from build123d import *
from build123d.topology import SkipClean

# Parameters (mm, degrees)
SKETCH_1_R      = 1.25
EXTRUDE_1_DEPTH = 2.5
FILLET_1_R      = 2
SKETCH_2_R      = 4.625
EXTRUDE_2_DEPTH = 13.7
SKETCH_3_R      = 1
EXTRUDE_3_DEPTH = 5.5
EXTRUDE_4_DEPTH = 2
EXTRUDE_START   = 11.3
SKETCH_5_R      = 13.75
EXTRUDE_5_DEPTH = 11.3
FILLET_2_R      = 4


with BuildPart() as part:
    # 草图1 → 凸台-拉伸1 (new body)
    with BuildSketch(Plane(origin=(0, 0, 0), x_dir=(1, 0, 0), z_dir=(0, 1, 0))):
        with BuildLine():
            Line((-1.948557159, 5.875), (-6.062177826, -1.25))
            ThreePointArc((-6.062177826, -1.25), (-8.010734985, -4.625), (-4.113620668, -4.625))
            Line((-4.113620668, -4.625), (4.113620668, -4.625))
            ThreePointArc((4.113620668, -4.625), (8.010734985, -4.625), (6.062177826, -1.25))
            Line((6.062177826, -1.25), (1.948557159, 5.875))
            ThreePointArc((1.948557159, 5.875), (0, 9.25), (-1.948557159, 5.875))
        make_face()
        with Locations(Location((0, 7, 0), (0, 0, 270))):
            Circle(SKETCH_1_R, mode=Mode.SUBTRACT)
        with Locations(Location((-6.062177826, -3.5, 0), (0, 0, 270))):
            Circle(SKETCH_1_R, mode=Mode.SUBTRACT)
        with Locations(Location((6.062177826, -3.5, 0), (0, 0, 270))):
            Circle(SKETCH_1_R, mode=Mode.SUBTRACT)
    extrude(amount=EXTRUDE_1_DEPTH)

    # 圆角1
    fillet_1_edges = [part.edges().sort_by_distance(p)[0] for p in [
        (-6.062177826, 1.25, 1.25),
        (-1.948557159, 1.25, -5.875),
        (1.948557159, 1.25, -5.875),
        (6.062177826, 1.25, 1.25),
        (4.113620668, 1.25, 4.625),
        (-4.113620668, 1.25, 4.625),
    ]]
    fillet(fillet_1_edges, radius=FILLET_1_R)

    # 草图2 → 凸台-拉伸2 (add)
    with BuildSketch(Plane(origin=(0, 2.5, 0), x_dir=(1, 0, 0), z_dir=(0, 1, 0))):
        with Locations(Location((0, 0, 0), (0, 0, 270))):
            Circle(SKETCH_2_R)
    extrude(amount=EXTRUDE_2_DEPTH)

    # 草图3 → 凸台-拉伸3 (add)
    with BuildSketch(Plane(origin=(0, 16.2, 0), x_dir=(1, 0, 0), z_dir=(0, 1, 0))):
        with Locations(Location((0, 0, 0), (0, 0, 270))):
            Circle(SKETCH_3_R)
    extrude(amount=EXTRUDE_3_DEPTH)

    # 草图4 → 凸台-拉伸4 (add)
    with BuildSketch(Plane(origin=(0, 16.2, 0), x_dir=(1, 0, 0), z_dir=(0, 1, 0))):
        with BuildLine():
            ThreePointArc((-3.6328125, -13.261416717), (0, -13.75), (3.6328125, -13.261416717))
            ThreePointArc((3.6328125, -13.261416717), (4.365393547, -9.060690569), (4.820970693, -4.820970693))
            ThreePointArc((4.820970693, -4.820970693), (9.060690569, -4.365393547), (13.261416717, -3.6328125))
            ThreePointArc((13.261416717, -3.6328125), (13.75, 0), (13.261416717, 3.6328125))
            ThreePointArc((13.261416717, 3.6328125), (9.060690569, 4.365393547), (4.820970693, 4.820970693))
            ThreePointArc((4.820970693, 4.820970693), (4.365393547, 9.060690569), (3.6328125, 13.261416717))
            ThreePointArc((3.6328125, 13.261416717), (0, 13.75), (-3.6328125, 13.261416717))
            ThreePointArc((-3.6328125, 13.261416717), (-4.365393547, 9.060690569), (-4.820970693, 4.820970693))
            ThreePointArc((-4.820970693, 4.820970693), (-9.060690569, 4.365393547), (-13.261416717, 3.6328125))
            ThreePointArc((-13.261416717, 3.6328125), (-13.75, 0), (-13.261416717, -3.6328125))
            ThreePointArc((-13.261416717, -3.6328125), (-9.060690569, -4.365393547), (-4.820970693, -4.820970693))
            ThreePointArc((-4.820970693, -4.820970693), (-4.365393547, -9.060690569), (-3.6328125, -13.261416717))
        make_face()
    extrude(amount=EXTRUDE_4_DEPTH)

    # 草图5 → 凸台-拉伸5 (add)
    with SkipClean():  # the faces are left unmerged after this step: merging them gives an invalid solid
        with BuildSketch(Plane.XZ.offset(-16.2).offset(EXTRUDE_START)):
            with Locations(Location((0, 0, 0), (0, 0, 270))):
                Circle(SKETCH_5_R)
        extrude(amount=-EXTRUDE_5_DEPTH)

    # 圆角2
    fillet_2_edges = [part.edges().sort_by_distance(p)[0] for p in [
        (-4.820970693, 17.2, 4.820970693),
        (4.820970693, 17.2, 4.820970693),
        (4.820970693, 17.2, -4.820970693),
        (-4.820970693, 17.2, -4.820970693),
    ]]
    fillet(fillet_2_edges, radius=FILLET_2_R)


solid = part.part
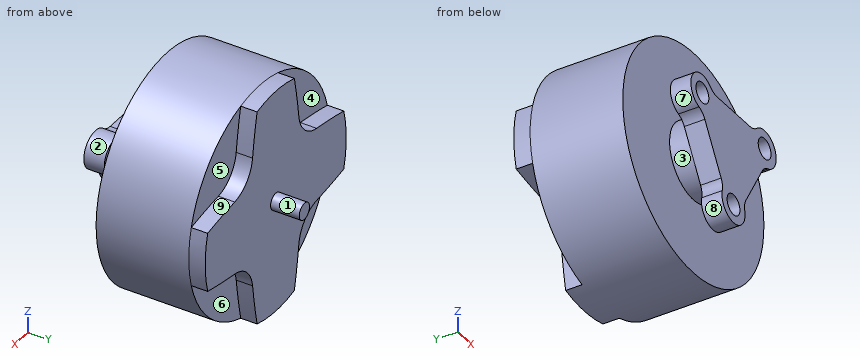
Read the model definition and answer for the solid it produces. Units are mm, in the model's axes. Face numbers are marked on the shaded views. A direction names the side the tool comes from. Give positions to 0.01 mm unless a question says otherwise; leave off trailing zeros. Write each loop counter-clockwise with the first axis right and the second up, starting at its lowest first coordinate (ties: lowest second). Pieces come first, ordered by that corner, then holes. Notation, with made-up numbers: M 46.25,-4.75 L 104.25,-4.75 A27 ccw 104.25,26.25 Z; hole C 58,19.5 d3. An arc over 180 degrees is marked long. One line per item, written item: value. Start each with the question number.
(1) A tool of negligible diameter and unlimited length cuts with its end or side. For the marked faces 1, 2, 3, 4 and 5, from which of +Z, -Z, +X, -X, +Y, -Y can it reach the whole face along a straight path? Write none if from no direction.
(2) Find section C-C (y = 5.75). Determine the outline of the cut face in (x, z).
(3) Find section B-B (z = -7). Give the number of separate pieces and of enclosed holes in the cut face, plus the area to 3 significant figures.
(4) Find the intervals of material crossed by line 1 (X direction, y = 0.9, z = 3.5); line 2 (X direction, y = 0.6, z = -7); line 3 (Y direction, x = -4.5, z = 5), in increasing order.
(5) Find section A-A (z = 0). Determine the outline of the cut face in (x, y) (3 decimals).
(6) Flat-ended cylindrical pins translate along their axes: pin 1 Ø10 at (y, z) = (3, -8) entering from -X; pin 2 Ø1 at (x, y) = (-3, 18.5) entering from +Z; pin 3 Ø2 at (x, y) = (9.5, 6.5) entering from +Z. Find the tip coordinate at first contact, or state that the pin passes through.
(7) Find section D-D (z = 10.75). Determine the outline of the cut face in (x, y).
(8) Determine the mould class of the marked faces 6, 7, 8 and 9 for opening direction X: pulls with the +X half, pulls with the -X half, needs draft (parallel to the pull), parting line crosses it, or undercut.
Results below:
1. face 1: +Y
1. face 2: -Y
1. face 3: none
1. face 4: +Z, -X, +Y
1. face 5: +Z, +X, +Y
2. outline: C 0,0 d27.5
3. separate pieces: 3
3. enclosed holes: 0
3. area: 292 mm^2
4. line 1: x = -8.31 to -7.31, -4.81 to 4.81, 7.31 to 8.31
4. line 2: x = -2.25 to -1.25, 1.25 to 2.25
4. line 3: y = 0 to 2.5, 4.9 to 18.2
5. outline: M -13.75,4.9 L -4.625,4.9 L -4.625,2.5 L -5.34,2.5 L -5.34,0 L 5.34,0 L 5.34,2.5 L 4.625,2.5 L 4.625,4.9 L 13.75,4.9 L 13.75,18.2 L 1,18.2 L 1,21.7 L -1,21.7 L -1,18.2 L -13.75,18.2 Z
6. pin 1: stops at x = -13.33
6. pin 2: stops at z = 13.5
6. pin 3: stops at z = 10.81
7. outline: M -8.57,4.9 L 8.57,4.9 L 8.57,16.2 L 4.1,16.2 L 4.1,18.2 L -4.1,18.2 L -4.1,16.2 L -8.57,16.2 Z
8. face 6: needs draft
8. face 7: undercut
8. face 8: parting line crosses it
8. face 9: pulls with the +X half
